from build123d import *

# Parameters (mm, degrees)
SKETCH_1_W          = 24
SKETCH_1_H          = 12
EXTRUDE_1_DEPTH     = 5
CUT_EXTRUDE_1_DEPTH = 15
SKETCH_2_3_R        = 2.5
EXTRUDE_2_DEPTH     = 1.5
SKETCH_4_R          = 2
EXTRUDE_3_DEPTH     = 1
EXTRUDE_4_DEPTH     = 9


with BuildPart() as part:
    # Sketch 1 → Extrude 1 (new, symmetric)
    with BuildSketch(Plane(origin=(0, 0, 0), x_dir=(1, 0, 0), z_dir=(0, 1, 0))):
        Rectangle(SKETCH_1_W, SKETCH_1_H)
    extrude(amount=EXTRUDE_1_DEPTH, both=True)

    # Sketch 2 → Cut-Extrude 1 (cut)
    with BuildSketch(Plane.ZY.offset(12)):
        with BuildLine():
            ThreePointArc((-6, 0), (-5.286764074, 2.837274331), (-3.31662479, 5))
            Line((-3.31662479, 5), (-6, 5))
            Line((-6, 5), (-6, 0))
        make_face()
        with BuildLine():
            Line((-6, -5), (-3.31662479, -5))
            ThreePointArc((-3.31662479, -5), (-5.286764074, -2.837274331), (-6, 0))
            Line((-6, 0), (-6, -5))
        make_face()
        with BuildLine():
            ThreePointArc((3.31662479, 5), (5.286764074, 2.837274331), (6, 0))
            Line((6, 0), (6, 5))
            Line((6, 5), (3.31662479, 5))
        make_face()
        with BuildLine():
            Line((6, -5), (6, 0))
            ThreePointArc((6, 0), (5.286764074, -2.837274331), (3.31662479, -5))
            Line((3.31662479, -5), (6, -5))
        make_face()
    extrude(amount=-CUT_EXTRUDE_1_DEPTH, mode=Mode.SUBTRACT)

    # Sketch 2_3 → Extrude 2 (add)
    with BuildSketch(Plane.ZY.offset(12)):
        with Locations(Location((0, 0, 0), (0, 0, 180))):
            Circle(SKETCH_2_3_R)
    extrude(amount=EXTRUDE_2_DEPTH)

    # Sketch 4 → Extrude 3 (add)
    with BuildSketch(Plane(origin=(12, 0, 0), x_dir=(0, 0, -1), z_dir=(1, 0, 0))):
        with Locations(Location((0, 0, 0), (0, 0, 180))):
            Circle(SKETCH_4_R)
    extrude(amount=EXTRUDE_3_DEPTH)

    # Sketch 5 → Extrude 4 (add)
    with BuildSketch(Plane(origin=(13, 0, 0), x_dir=(0, 0, -1), z_dir=(1, 0, 0))):
        with BuildLine():
            Line((1.118033989, 1), (-1.118033989, 1))
            ThreePointArc((-1.118033989, 1), (-0.535233135, -1.401258538), (1.5, 0))
            ThreePointArc((1.5, 0), (1.401258538, 0.535233135), (1.118033989, 1))
        make_face()
    extrude(amount=EXTRUDE_4_DEPTH)


solid = part.part
Read the model definition and answer for the solid it produces. Units are mm, in the model's axes. A direction names the side the tool comes from. Give positions to 0.01 mm unless a question says otherwise; leave off trailing zeros. Write each loop counter-clockwise with the first axis right and the second up, starting at its lowest first coordinate (ties: lowest second). Pieces come first, ordered by that corner, then holes. Notation, with made-up numbers: (61, 23) - (105, 23) arc R14 cw to (105, 49) - close; hole circle Ø2 at (25, 33.25). An arc over 180 degrees is marked (long way). Answer in a Markdown table with one row per item. Add a question column.
Item 1: A tool of negligible diameter and unlimited length cuts with its end or side. For faces 1 (the face through (3, -4, -5)), 2 (the face through (17, 1, 0)), 3 (the face through (12.493, 1.952, -0.434)), from which of +Z, -Z, +X, -X, +Y, -Y can it reach the whole face along a straight path? Write none if from no direction.
Item 2: Section A-A, the plane x = 1.5 is taken. Write down the section's boundary in (y, z).
Item 3: Section D-D, the plane z = 5 is taken. Write down the section's boundary in (x, y).
Item 4: Section C-C, the plane y = 4.25 is taken. Write down the section's boundary in (x, z), and give its area (3 significant figures).
Item 5: Flat-ended cylindrical pins translate along their axes: P1, Ø1.3, axis at y = 3, z = -4, coming from the -X side; P2, Ø0.7, axis at x = 15.5, z = 0.5, coming from the +Y side; P3, Ø5, axis at y = -0.5, z = 2.5, coming from the +X side. Find the tip coordinate at first contact, or state that the pin passes through.
Item 6: Find the intervals of material crossed by L1, parallel to X at y = -2.5, z = -0.5; L2, parallel to Y at x = -8, z = -5; L3, parallel to X at y = 1.5, z = 1.25, in increasing order.
Item 7: Section B-B, the plane z = 0 is taken. Write down the section's boundary in (x, y).
Recorded:
| question | item | result |
|---|---|---|
| 1 | face 1 | -Z, -X, -Y |
| 1 | face 2 | +Z, -Z, +X, +Y |
| 1 | face 3 | +X |
| 2 | outline | (-5, -3.32) arc R6 ccw to (5, -3.32) - (5, 3.32) arc R6 ccw to (-5, 3.32) - close |
| 3 | outline | (-12, -3.32) - (3, -3.32) - (3, -5) - (12, -5) - (12, 5) - (3, 5) - (3, 3.32) - (-12, 3.32) - close |
| 4 | outline | (-12, -4.24) - (3, -4.24) - (3, -6) - (12, -6) - (12, 6) - (3, 6) - (3, 4.24) - (-12, 4.24) - close |
| 4 | area | 235 mm2 |
| 5 | P1 | stops at x = -12 |
| 5 | P2 | stops at y = 1 |
| 5 | P3 | stops at x = 22 |
| 6 | L1 | x = -12 to 12 |
| 6 | L2 | y = -3.32 to 3.32 |
| 6 | L3 | x = -13.5 to 13 |
| 7 | outline | (-13.5, -2.5) - (-12, -2.5) - (-12, -5) - (12, -5) - (12, -2) - (13, -2) - (13, -1.5) - (22, -1.5) - (22, 1) - (13, 1) - (13, 2) - (12, 2) - (12, 5) - (-12, 5) - (-12, 2.5) - (-13.5, 2.5) - close |
